```python
from build123d import *

# Parameters (mm, degrees)
SKETCH_2_R          = 41.5
CUT_EXTRUDE_1_DEPTH = 13
SKETCH_3_R          = 6.5
CUT_EXTRUDE_2_DEPTH = 65.097581858
SKETCH_4_R          = 7.5
SKETCH_4_R_2        = 6.5
EXTRUDE_1_DEPTH     = 22.6
M3X0_51_D           = 2.5
FILLET_1_R          = 1
SKETCH_8_R          = 41.5
SKETCH_8_R_2        = 7.5
EXTRUDE_2_DEPTH     = 7.5


with BuildPart() as part:
    # Эскиз1 → Повернуть1 (revolve)
    with BuildSketch(Plane(origin=(0, 0, 0), x_dir=(1, 0, 0), z_dir=(0, 1, 0))):
        Polygon((0, 0), (-43.5, 0), (-43.5, 15), (-20, 18), (0, 18), align=None)
    revolve(axis=Axis((0, 0, -18), (0, 0, 1)))

    # Эскиз2 → Вырез-Вытянуть1 (cut)
    with BuildSketch(Plane.XY):
        Circle(SKETCH_2_R)
    extrude(amount=-CUT_EXTRUDE_1_DEPTH, mode=Mode.SUBTRACT)

    # Эскиз3 → Вырез-Вытянуть2 (cut, through all)
    with BuildSketch(Plane(origin=(0, 0, -18), x_dir=(-1, 0, 0), z_dir=(0, 0, -1))):
        Circle(SKETCH_3_R)
    extrude(amount=-CUT_EXTRUDE_2_DEPTH, mode=Mode.SUBTRACT)

    # Эскиз4 → Бобышка-Вытянуть1 (add)
    with BuildSketch(Plane.XY.offset(-13)):
        Circle(SKETCH_4_R)
        with Locations(Location((0, 0, 0), (0, 0, 180))):
            Circle(SKETCH_4_R_2, mode=Mode.SUBTRACT)
    extrude(amount=EXTRUDE_1_DEPTH)

    # Отверстие обработанное метчиком M3x0.51 (through all)
    with Locations(Plane(origin=(0, 0, -18), x_dir=(-1, 0, 0), z_dir=(0, 0, -1))):
        with Locations((-12.374368671, 12.374368671), (0, 17.5), (12.374368671, 12.374368671), (17.5, 0), (12.374368671, -12.374368671), (0, -17.5), (-12.374368671, -12.374368671), (-17.5, 0), (-12.5, 0), (0, 12.5), (12.5, 0), (0, -12.5)):
            Hole(M3X0_51_D / 2)

    # Скругление1
    fillet_1_edges = [part.edges().sort_by_distance(p)[0] for p in [
        (20, 0, -18),
        (43.5, 0, -15),
    ]]
    fillet(fillet_1_edges, radius=FILLET_1_R)

    # Эскиз8 → Бобышка-Вытянуть2 (add)
    with BuildSketch(Plane.XY.offset(-13)):
        Circle(SKETCH_8_R)
        Circle(SKETCH_8_R_2, mode=Mode.SUBTRACT)
    extrude(amount=EXTRUDE_2_DEPTH)


solid = part.part
```
Source: CAD feature listing. Evaluate the final solid. Frame: model axes, mm. A direction names the side the tool comes from. Round coordinates to 2 decimals unless told otherwise and drop trailing zeros. Loops run counter-clockwise (first coordinate to the right, second up) from the corner with the lowest first, then second, coordinate; pieces in that order, holes last. Notation, with made-up numbers: M 60.5,42 L 69.5,42 A15 cw 69.5,59 Z; hole C 4,-12.75 d4. An arc over 180 degrees is marked long. Use a Markdown table: item, result. Add a question column.
1. Cut plane A-A, the plane z = -10.5. Output: boundary loops of the cut face in (x, y).
2. Pull-direction query (Y, two-part tool) for faces 1 (the flat face through (38.5, 15.9, 0)), 2 (the flat face through (0, 13, -13)), 3 (the conical face through (-20.182, -6.355, -17.852)), 4 (the cylindrical face through (-13.75, 0.05, -15.47)); classes: +Y half, -Y half, draft (parallel to the pull), parting line (faces both ways), or undercut.
3. Set-up query: faces 5 (the cylindrical face through (5.158, 3.955, -4.393)), 6 (the cylindrical face through (-11.7, -11.32, -15.47)). Return all of +Z, -Z, +X, -X, +Y, -Y with unobstructed straight access to the full face (end or side cutting, diameter ignored); none if empty.
4. Cut plane B-B, the plane z = 2. Output: boundary loops of the cut face in (x, y).
5. Contact query for flat-ended pins moving along their axis: pin 1 (4 mm diameter, centred on y = -6.5, z = 1, fed in from +X); pin 2 (2 mm diameter, centred on x = 0, y = -12.5, fed in from +Z); pin 3 (12 mm diameter, centred on x = -2, z = 7, fed in from -Y). Output: stop coordinate, or through.
6. Ray query, line 1 along X through (y, z) = (3.5, -3.75); line 2 along X through (y, z) = (-24, -2); line 3 along X through (y, z) = (-17.5, -1). Return the intervals inside material, ascending. Write a range as [from, to].
Solution:
| question | item | result |
|---|---|---|
| 1 | outline | C 0,0 d87; hole C 0,0 d13 |
| 2 | face 1 | draft |
| 2 | face 2 | undercut |
| 2 | face 3 | parting line |
| 2 | face 4 | undercut |
| 3 | face 5 | +Z, -Z |
| 3 | face 6 | -Z |
| 4 | outline | C 0,0 d15; hole C 0,0 d13 |
| 5 | pin 1 | stops at x = 43.24 |
| 5 | pin 2 | stops at z = -5.5 |
| 5 | pin 3 | stops at y = -7.5 |
| 6 | line 1 | x = [-43.36, -41.35], [-6.63, -5.48], [5.48, 6.63], [41.35, 43.36] |
| 6 | line 2 | x = [-36.28, -33.86], [33.86, 36.28] |
| 6 | line 3 | x = [-39.82, -37.63], [37.63, 39.82] |
